Geometry: final body of the model. Coordinates: model frame, mm. A direction names the side the tool comes from. Coordinates: 2 decimals unless noted, no trailing zeros. Write each loop counter-clockwise with the first axis right and the second up, starting at its lowest first coordinate (ties: lowest second). Pieces come first, ordered by that corner, then holes.
Autodesk Inventor part; units mm, degrees
ref_plane "YZ Plane" through (0, 0, 0) normal (1, 0, 0) x (0, 1, 0)
ref_plane "XZ Plane" through (0, 0, 0) normal (0, 1, 0) x (-1, 0, 0)
ref_plane "XY Plane" through (0, 0, 0) normal (0, 0, 1) x (1, 0, 0)
sketch "Sketch1" plane through (0, 0, 0) normal (0, 1, 0) x (-1, 0, 0)
  line L0 (0, 0) -> (426.7814, 0) construction
  line L1 (426.7814, 0) -> (426.7814, -191.0355) construction
  line L2 (426.7814, -191.0355) -> (0, -191.0355) construction
  line L3 (0, -191.0355) -> (0, 0) construction
  line L4 (332.8385, -18.2414) -> (332.8385, -25.9274)
  line L5 (332.8385, -25.9274) -> (308.3392, -25.9274)
  line L6 (308.3392, -25.9274) -> (308.3392, -33.9978)
  line L7 (308.3392, -33.9978) -> (300.0767, -33.9978)
  line L8 (300.0767, -33.9978) -> (300.0767, -59.1696)
  line L9 (300.0767, -59.1696) -> (324.672, -59.1696)
  line L10 (324.672, -59.1696) -> (324.672, -66.3753)
  line L11 (324.672, -66.3753) -> (316.3135, -66.3753)
  line L12 (316.3135, -66.3753) -> (316.3135, -72.5241)
  line L13 (316.3135, -72.5241) -> (314.6458, -72.5241)
  line L14 (314.6458, -72.5241) -> (314.6458, -74.979)
  line L15 (314.6458, -74.979) -> (300.5812, -74.979)
  line L16 (300.5812, -74.979) -> (300.5812, -83.958)
  line L17 (300.5812, -83.958) -> (317.2389, -83.958)
  line L18 (317.2389, -83.958) -> (317.2389, -77.9978)
  line L19 (317.2389, -77.9978) -> (319.6927, -77.9978)
  line L20 (319.6927, -77.9978) -> (319.6927, -75.753)
  line L21 (319.6927, -75.753) -> (333.8192, -75.753)
  line L22 (333.8192, -75.753) -> (333.8192, -67.5016)
  line L23 (333.8192, -67.5016) -> (338.8738, -67.5016)
  line L24 (338.8738, -67.5016) -> (338.8738, -69.7696)
  line L25 (338.8738, -69.7696) -> (340.7167, -69.7696)
  line L26 (340.7167, -69.7696) -> (340.7167, -75.5985)
  line L27 (349.6517, -59.1696) -> (342.2405, -59.1696)
  line L28 (342.2405, -59.1696) -> (342.2405, -64.5393)
  line L29 (342.2405, -64.5393) -> (343.8251, -64.5393)
  line L30 (343.8251, -64.5393) -> (343.8251, -66.7322)
  line L31 (343.8251, -66.7322) -> (349.6517, -66.7322)
  line L32 (325.5834, -43.5764) -> (325.5834, -50.3454)
  line L33 (325.5834, -50.3454) -> (340.7167, -50.3454)
  line L34 (340.7167, -50.3454) -> (340.7167, -43.5764)
  line L35 (340.7167, -43.5764) -> (325.5834, -43.5764)
  line L36 (340.7167, -75.5985) -> (349.6517, -75.5985)
  line L37 (332.8385, -18.2414) -> (349.6517, -18.2414)
  line L38 (366.4649, -18.2414) -> (366.4649, -25.9274)
  line L39 (366.4649, -25.9274) -> (390.9642, -25.9274)
  line L40 (390.9642, -25.9274) -> (390.9642, -33.9978)
  line L41 (390.9642, -33.9978) -> (399.2267, -33.9978)
  line L42 (399.2267, -33.9978) -> (399.2267, -59.1696)
  line L43 (399.2267, -59.1696) -> (374.6314, -59.1696)
  line L44 (374.6314, -59.1696) -> (374.6314, -66.3753)
  line L45 (374.6314, -66.3753) -> (382.9899, -66.3753)
  line L46 (382.9899, -66.3753) -> (382.9899, -72.5241)
  line L47 (382.9899, -72.5241) -> (384.6575, -72.5241)
  line L48 (384.6575, -72.5241) -> (384.6575, -74.979)
  line L49 (384.6575, -74.979) -> (398.7222, -74.979)
  line L50 (398.7222, -74.979) -> (398.7222, -83.958)
  line L51 (398.7222, -83.958) -> (382.0645, -83.958)
  line L52 (382.0645, -83.958) -> (382.0645, -77.9978)
  line L53 (382.0645, -77.9978) -> (379.6107, -77.9978)
  line L54 (379.6107, -77.9978) -> (379.6107, -75.753)
  line L55 (379.6107, -75.753) -> (365.4842, -75.753)
  line L56 (365.4842, -75.753) -> (365.4842, -67.5016)
  line L57 (365.4842, -67.5016) -> (360.4296, -67.5016)
  line L58 (360.4296, -67.5016) -> (360.4296, -69.7696)
  line L59 (360.4296, -69.7696) -> (358.5867, -69.7696)
  line L60 (358.5867, -69.7696) -> (358.5867, -75.5985)
  line L61 (349.6517, -59.1696) -> (357.0629, -59.1696)
  line L62 (357.0629, -59.1696) -> (357.0629, -64.5393)
  line L63 (357.0629, -64.5393) -> (355.4783, -64.5393)
  line L64 (355.4783, -64.5393) -> (355.4783, -66.7322)
  line L65 (355.4783, -66.7322) -> (349.6517, -66.7322)
  line L66 (373.72, -43.5764) -> (373.72, -50.3454)
  line L67 (373.72, -50.3454) -> (358.5867, -50.3454)
  line L68 (358.5867, -50.3454) -> (358.5867, -43.5764)
  line L69 (358.5867, -43.5764) -> (373.72, -43.5764)
  line L70 (358.5867, -75.5985) -> (349.6517, -75.5985)
  line L71 (366.4649, -18.2414) -> (349.6517, -18.2414)
  dimension "d24" = 25.5068
extrude "Extrusion1" add sketch "Sketch1" along normal blind 6.35
properties part number "Monster5"
Item 1: Set-up query: faces 4 (the flat face through (-357.063, 3, -62)), 5 (the flat face through (-374.631, 3, -63)), 6 (the flat face through (-395, 3, -33.998)). Return all of +Z, -Z, +X, -X, +Y, -Y with unobstructed straight access to the full face (end or side cutting, diameter ignored); none if empty.
Derived:
face 4: +Y, -Y
face 5: -X, +Y, -Y
face 6: +Z, -X, +Y, -Y
Item 2: Section A-A, the plane x = -372. Output: boundary loops of the cut face in (y, z), plus the area to 3 significant figures.
Derived:
outline: (0, -75.75) - (6.35, -75.75) - (6.35, -50.35) - (0, -50.35) - close; (0, -43.58) - (6.35, -43.58) - (6.35, -25.93) - (0, -25.93) - close
area: 273 mm2
Item 3: Pull-direction query (Z, two-part tool) for faces 1 (the flat face through (-309, 3, -83.958)), 2 (the flat face through (-349, 0, -51)), 3 (the flat face through (-316.314, 3, -69)); classes: released by +Z, released by -Z, zero draft, split by the parting line, or undercut.
Derived:
face 1: released by -Z
face 2: zero draft
face 3: undercut
Item 4: Material intervals for probe 1 along Z at (x, y) = (-312, 5.25); probe 2 along Z at (x, y) = (-338, 1.25); probe 3 along X at (y, z) = (4.25, -69), sorted ascending.
Derived:
probe 1: z = -83.96 to -74.98, -59.17 to -25.93
probe 2: z = -67.5 to -50.35, -43.58 to -18.24
probe 3: x = -382.99 to -365.48, -360.43 to -338.87, -333.82 to -316.31
Item 5: Pin query (flat end, axial travel): pin 1 (1.9 mm diameter, centred on x = -331.5, y = 4.5, fed in from +Z); pin 2 (3 mm diameter, centred on y = 3, z = -71.5, fed in from -X); pin 3 (2 mm diameter, centred on x = -389, z = -25.5, fed in from -Y); pin 4 (1 mm diameter, centred on x = -363, z = -49, fed in from +Y). Return the tip coordinate at first contact, or that it passes through.
Derived:
pin 1: stops at z = -25.93
pin 2: stops at x = -384.66
pin 3: stops at y = 0
pin 4: passes through
Item 6: Section B-B, the plane z = -63. Output: boundary loops of the cut face in (x, y).
Derived:
outline: (-374.63, 0) - (-357.06, 0) - (-357.06, 6.35) - (-374.63, 6.35) - close; (-342.24, 0) - (-324.67, 0) - (-324.67, 6.35) - (-342.24, 6.35) - close
Item 7: Section C-C, the plane z = -45.5. Output: boundary loops of the cut face in (x, y).
Derived:
outline: (-399.23, 0) - (-373.72, 0) - (-373.72, 6.35) - (-399.23, 6.35) - close; (-358.59, 0) - (-340.72, 0) - (-340.72, 6.35) - (-358.59, 6.35) - close; (-325.58, 0) - (-300.08, 0) - (-300.08, 6.35) - (-325.58, 6.35) - close
Item 8: Section D-D, the plane y = 4.75. State how many separate pieces and enclosed holes the cut face has, plus the area to 3 significant figures.
Derived:
separate pieces: 1
enclosed holes: 3
area: 4,300 mm2
